CAD build for the part. Positions are in the model's coordinates, mm. A direction names the side the tool comes from. Coordinates: 2 decimals unless noted, no trailing zeros. Write each loop counter-clockwise with the first axis right and the second up, starting at its lowest first coordinate (ties: lowest second). Pieces come first, ordered by that corner, then holes.
```python
from build123d import *

# Parameters (mm, degrees)
SKETCH_1_W          = 29
SKETCH_1_H          = 29
EXTRUDE_1_DEPTH     = 1
SKETCH_2_W          = 31
SKETCH_2_H          = 31
SKETCH_2_W_2        = 29
SKETCH_2_H_2        = 29
EXTRUDE_2_DEPTH     = 13
EXTRUDE_4_DEPTH     = 5
CUT_EXTRUDE_START   = -14
CUT_EXTRUDE_2_DEPTH = 27
SKETCH_5_R          = 2.15366908
EXTRUDE_5_DEPTH     = 1
FILLET_2_R          = 2
FILLET_3_R          = 1.5
SKETCH_6_R          = 1.5
CUT_EXTRUDE_3_DEPTH = 10
SKETCH_7_RX         = 3.115871069
SKETCH_7_RY         = 2.3606007
EXTRUDE_6_DEPTH     = 1


with BuildPart() as part:
    # Sketch 1 → Extrude 1 (new body)
    with BuildSketch(Plane.XY):
        Rectangle(SKETCH_1_W, SKETCH_1_H)
        Polygon((-11.5, 0), (-11.5, 9.5), (11.5, 9.5), (11.5, -5.5), (-11.5, -5.5), align=None, mode=Mode.SUBTRACT)
    extrude(amount=EXTRUDE_1_DEPTH)

    # Sketch 2 → Extrude 2 (add)
    with BuildSketch(Plane.XY.offset(1)):
        Rectangle(SKETCH_2_W, SKETCH_2_H)
        Rectangle(SKETCH_2_W_2, SKETCH_2_H_2, mode=Mode.SUBTRACT)
    extrude(amount=-EXTRUDE_2_DEPTH)

    # Sketch 3 → Extrude 4 (add)
    with BuildSketch(Plane(origin=(15.5, 0, 0), x_dir=(0, 0, -1), z_dir=(1, 0, 0))):
        with BuildLine():
            Line((1.684082639, 8.989995997), (0.397094894, -5.595641246))
            Line((0.397094894, -5.595641246), (10.451208148, -10.79214922))
            Line((10.451208148, -10.79214922), (9.295909354, 8.989995997))
            ThreePointArc((9.295909354, 8.989995997), (5.489995997, 12.795909354), (1.684082639, 8.989995997))
        make_face()
    extrude_4 = extrude(amount=EXTRUDE_4_DEPTH)

    # Sketch 4 → Cut-Extrude 2 (cut)
    with BuildSketch(Plane(origin=(0, -0.077997079, -0.883953322), x_dir=(1, 0, 0), z_dir=(0, 0.08789514896151537, 0.9961297319069606)).offset(CUT_EXTRUDE_START)):
        Polygon((18, 9.103224997), (20.5, -9.831770213), (20.5, 13.243659675), (18, 13.243659675), align=None)
    cut_extrude_2 = extrude(amount=CUT_EXTRUDE_2_DEPTH, mode=Mode.SUBTRACT)

    # Sketch 5 → Extrude 5 (add)
    with BuildSketch(Plane(origin=(18, 0, 0), x_dir=(0, 0, -1), z_dir=(1, 0, 0))):
        with Locations(Location((5.489995997, 8.989995997, 0), (0, 0, 183.893189549))):
            Circle(SKETCH_5_R)
    extrude_5 = extrude(amount=EXTRUDE_5_DEPTH)

    # Mirror 1: Extrude 4, Cut-Extrude 2, Extrude 5 across plane
    add(extrude_4.mirror(Plane(origin=(0, 0, 0), x_dir=(0, 0, 1), z_dir=(1, 0, 0))))
    add(cut_extrude_2.mirror(Plane(origin=(0, 0, 0), x_dir=(0, 0, 1), z_dir=(1, 0, 0))), mode=Mode.SUBTRACT)
    add(extrude_5.mirror(Plane(origin=(0, 0, 0), x_dir=(0, 0, 1), z_dir=(1, 0, 0))))

    # Fillet 2
    fillet_2_edges = [part.edges().sort_by_distance(p)[0] for p in [
        (15.5, -15.5, -5.5),
        (-15.5, -15.5, -5.5),
        (-15.5, 15.5, -5.5),
        (15.5, 15.5, -5.5),
    ]]
    fillet(fillet_2_edges, radius=FILLET_2_R)

    # Fillet 3
    fillet_3_edges = [part.edges().sort_by_distance(p)[0] for p in [
        (-18, -10.79214922, -10.451208148),
        (-17.716616755, -5.595641246, -0.397094894),
        (18, -10.79214922, -10.451208148),
        (17.716616755, -5.595641246, -0.397094894),
    ]]
    fillet(fillet_3_edges, radius=FILLET_3_R)

    # Sketch 6 → Cut-Extrude 3 (cut)
    with BuildSketch(Plane(origin=(0, -14.5, 0), x_dir=(1, 0, 0), z_dir=(0, 1, 0))):
        with Locations(Location((0, 8.292466775, 0), (0, 0, 270))):
            Circle(SKETCH_6_R)
    extrude(amount=-CUT_EXTRUDE_3_DEPTH, mode=Mode.SUBTRACT)

    # Sketch 7 → Extrude 6 (add)
    # profile 1 of 3: a face of its own
    with BuildSketch(Plane.XY.offset(1)):
        Polygon((-14.13707497, -6.569596288), (-12.29339398, -6.569596288), (-9.531936558, -9.999148248), (-6.993177314, -6.569596288), (-5.148542266, -6.569596288), (-8.282186736, -10.802765134), (-4.967091233, -14.230413654), (-7.35222414, -14.230413654), (-9.483652502, -11.583317139), (-12.183939304, -14.230413654), (-13.406884876, -14.230413654), (-10.757959228, -11.129248682), align=None)
    # profile 2 of 3: a face of its own
    with BuildSketch(Plane.XY.offset(1)):
        Polygon((-3.07368936, -6.569596288), (3.518176746, -6.569596288), (3.518176746, -8.181354333), (-1.127695874, -13.161462393), (3.518176746, -13.161462393), (3.518176746, -14.230413654), (-3.60816499, -14.230413654), (2.458193197, -7.72762682), (-3.07368936, -7.72762682), align=None)
    # profile 3 of 3: a face of its own
    with BuildSketch(Plane.XY.offset(1)):
        with BuildLine():
            add(Edge.make_bspline(
                [(13.257578349, -13.064625962), (16.352824865, -7.664798791), (10.641635787, -6.629296303), (4.930446709, -5.593793814), (6.299215158, -11.802996851), (7.667983606, -18.012199887), (12.309307415, -14.194426658)],
                knots=[1.006525836, 1.006525836, 1.006525836, 2.978836938, 2.978836938, 4.95114804, 4.95114804, 6.923459142, 6.923459142, 6.923459142], degree=2, weights=[1, 0.551899857, 1, 0.551899857, 1, 0.551899857, 1]))
            add(Edge.make_bspline(
                [(12.309307415, -14.194426658), (13.611329655, -15.324791628), (14.10540557, -14.736133584), (14.599481485, -14.147475541), (13.257578349, -13.064625962)],
                knots=[4.671290612, 4.671290612, 4.671290612, 6.282456981, 6.282456981, 7.89362335, 7.89362335, 7.89362335], degree=2, weights=[1, 0.69269074, 1, 0.69269074, 1]))
        make_face()
        with Locations(Location((10.02096358, -10.802765134), (0, 0, -90))):
            Ellipse(SKETCH_7_RX, SKETCH_7_RY, mode=Mode.SUBTRACT)
    extrude(amount=EXTRUDE_6_DEPTH)


solid = part.part
```
Item 1: Saw through at C-C, the plane y = 10. Write the cut outline in (x, z).
Item 2: Saw through at A-A, the plane x = 0. Write the cut outline in (y, z), and give its area (3 significant figures).
Item 3: Wall check: line 1 along Y through (x, z) = (-7, -8); line 2 along Y through (x, z) = (-6, 0.75). Give the ranges that are in metal, low to high.
Item 4: Flat gauge pins, fed straight in: pin 1 Ø0.5 at (y, z) = (-14, 1.5) entering from +X; pin 2 Ø0.8 at (x, z) = (-6, 1.5) entering from +Y; pin 3 Ø4 at (x, y) = (3, -4.5) entering from -Z. Where does each tip first touch, or does it go through?
Item 5: Two-plate mould, pull along Y, no slides. Class faces 1 (the flat face through (-0.3, -7.728, 1.5)), 2 (the flat face through (12.3, -12.2, 2)), 3 (the flat face through (-8.4, -12.93, 1.49)): +Y half, -Y half, draft (parallel to the pull), parting line (faces both ways), or undercut.
Item 6: Saw through at D-D, the plane y = 3. Write the cut outline in (x, z), and give its area (3 significant figures).
Item 7: Which spindle directions (+Z, -Z, +X, -X, +Y, -Y) get a long thin tool onto all of the face, cutting with end or side? Do faces 4 (the flat face through (-14.5, 0, -6)), 5 (the flat face through (-13.2, -6.57, 1.5)), 6 (the flat face through (-6.693, -8.657, 1.493)), 7 (the flat face through (-17.9, -7.796, -4.653)). Say none if no direction does.
Item 8: Saw through at B-B, the plane z = -2.5. Write the cut outline in (x, y).
Working result:
1. outline: (-19, -7.39) - (-18, -7.39) - (-18, -9.16) - (-15.5, -9.16) - (-15.5, -12) - (-14.5, -12) - (-14.5, 0) - (14.5, 0) - (14.5, -12) - (15.5, -12) - (15.5, -9.16) - (18, -9.16) - (18, -7.39) - (19, -7.39) - (19, -3.59) - (18, -3.59) - (18, -1.82) - (15.5, -1.82) - (15.5, 1) - (-15.5, 1) - (-15.5, -1.82) - (-18, -1.82) - (-18, -3.59) - (-19, -3.59) - close
2. outline: (-15.5, -12) - (-14.5, -12) - (-14.5, -9.79) - (-15.5, -9.79) - close; (-15.5, -6.79) - (-14.5, -6.79) - (-14.5, 0) - (-5.5, 0) - (-5.5, 1) - (-6.57, 1) - (-6.57, 2) - (-7.73, 2) - (-7.73, 1) - (-10.36, 1) - (-10.36, 2) - (-11.95, 2) - (-11.95, 1) - (-13.16, 1) - (-13.16, 2) - (-14.23, 2) - (-14.23, 1) - (-15.5, 1) - close; (9.5, 0) - (14.5, 0) - (14.5, -12) - (15.5, -12) - (15.5, 1) - (9.5, 1) - close
2. area: 40.8 mm2
3. line 1: y = -15.5 to -14.5, 14.5 to 15.5
3. line 2: y = -15.5 to -5.5, 9.5 to 15.5
4. pin 1: stops at x = 14.16
4. pin 2: stops at y = -6.57
4. pin 3: stops at z = 0
5. face 1: undercut
5. face 2: draft
5. face 3: -Y half
6. outline: (-18.79, -1.16) - (-18.7, -9.65) - (-15.5, -9.65) - (-15.5, -12) - (-14.5, -12) - (-14.5, 0) - (-11.5, 0) - (-11.5, 1) - (-15.5, 1) - (-15.5, -1.16) - close; (11.5, 0) - (14.5, 0) - (14.5, -12) - (15.5, -12) - (15.5, -9.65) - (18.7, -9.65) - (18.79, -1.16) - (15.5, -1.16) - (15.5, 1) - (11.5, 1) - close
6. area: 87.1 mm2
7. face 4: -Z
7. face 5: +Z, +X, -X, +Y
7. face 6: +Z
7. face 7: +Z, -X, -Y
8. outline: (-20.05, -6.68) - (-15.5, -6.68) - (-15.5, -13.5) arc R2 ccw to (-13.5, -15.5) - (13.5, -15.5) arc R2 ccw to (15.5, -13.5) - (15.5, -6.68) - (20.05, -6.68) - (18, 8.92) - (18, 11.34) - (15.5, 11.34) - (15.5, 13.5) arc R2 ccw to (13.5, 15.5) - (-13.5, 15.5) arc R2 ccw to (-15.5, 13.5) - (-15.5, 11.34) - (-18, 11.34) - (-18, 8.92) - close; hole (-14.5, -14.5) - (14.5, -14.5) - (14.5, 14.5) - (-14.5, 14.5) - close
